from build123d import *

# Parameters (mm, degrees)
F1_DEPTH = 2.5
F2_W     = 133
F2_H     = 133
F3_DEPTH = 5.001
F4_SIZE  = 1


with BuildPart() as f1:
    # F0 (on Top) → F1 (new body, symmetric)
    with BuildSketch(Plane.XY):
        Polygon((-207, 415), (-223, -415), (223, -415), (223, 415), align=None)
    extrude(amount=F1_DEPTH, both=True)

    # F2 (on face) → F3 (cut, through all)
    with BuildSketch(Plane.XY.offset(2.5)):
        with Locations((-57.5, -310.5)):
            Rectangle(F2_W, F2_H)
    extrude(amount=-F3_DEPTH, mode=Mode.SUBTRACT)

    # F4
    f4_edges = [f1.edges().sort_by_distance(p)[0] for p in [
        (-215, 0, 2.5),
        (-215, 0, -2.5),
        (8, 415, 2.5),
        (8, 415, -2.5),
        (223, 0, 2.5),
        (223, 0, -2.5),
        (0, -415, 2.5),
        (0, -415, -2.5),
    ]]
    chamfer(f4_edges, length=F4_SIZE)


solid = f1.part
The listing builds one solid part. Answer for the finished solid, in the listing's coordinates (mm). Coordinates: 2 decimals unless noted, no trailing zeros. Loops run counter-clockwise (first coordinate to the right, second up) from the corner with the lowest first, then second, coordinate; pieces in that order, holes last.
1) Find the intervals of material crossed by L1, parallel to Y at x = -76.5, z = 1.55; L2, parallel to Y at x = -92, z = -1.8; L3, parallel to X at y = -347.5, z = 1.85, in increasing order.
2) Find section B-B on z = -0.3. Write down the section's boundary in (x, y), then the cut area to 3 significant figures.
3) Flat-ended cylindrical pins translate along their axes: pin 1 Ø1.5 at (y, z) = (-331, 1) entering from -X; pin 2 Ø2 at (y, z) = (277, 0) entering from -X. Find the tip coordinate at first contact, or state that the pin passes through.
4) Find section D-D on y = 119. Write down the section's boundary in (x, z), then the cut area to 3 significant figures.
5) Find section C-C on y = -301. Write down the section's boundary in (x, z), then the cut area to 3 significant figures.
6) Find section A-A on x = -8.5. Write down the section's boundary in (y, z), then the cut area to 3 significant figures.
Values:
1. L1: y = -414.95 to -377, -244 to 414.95
1. L2: y = -414.7 to -377, -244 to 414.7
1. L3: x = -221.35 to -124, 9 to 222.65
2. outline: (-223, -415) - (223, -415) - (223, 415) - (-207, 415) - close; hole (-124, -377) - (9, -377) - (9, -244) - (-124, -244) - close
2. area: 346,000 mm2
3. pin 1: stops at x = -221.4
3. pin 2: stops at x = -209.68
4. outline: (-212.71, -1.5) - (-211.71, -2.5) - (222, -2.5) - (223, -1.5) - (223, 1.5) - (222, 2.5) - (-211.71, 2.5) - (-212.71, 1.5) - close
4. area: 2,180 mm2
5. outline: (-220.8, -1.5) - (-219.8, -2.5) - (-124, -2.5) - (-124, 2.5) - (-219.8, 2.5) - (-220.8, 1.5) - close; (9, -2.5) - (222, -2.5) - (223, -1.5) - (223, 1.5) - (222, 2.5) - (9, 2.5) - close
5. area: 1,550 mm2
6. outline: (-415, -1.5) - (-414, -2.5) - (-377, -2.5) - (-377, 2.5) - (-414, 2.5) - (-415, 1.5) - close; (-244, -2.5) - (414, -2.5) - (415, -1.5) - (415, 1.5) - (414, 2.5) - (-244, 2.5) - close
6. area: 3,480 mm2
